Geometry check sheet. Reference: the model listing, model coordinates, mm. A direction names the side the tool comes from. Give positions to 0.01 mm unless a question says otherwise; leave off trailing zeros. Loops run counter-clockwise (first coordinate to the right, second up) from the corner with the lowest first, then second, coordinate; pieces in that order, holes last. Notation, with made-up numbers: (-17.75, 75) -> (-9.75, 75) arc R4 ccw to (-9.75, 82) -> close; hole circle Ø5 at (45, 63). An arc over 180 degrees is marked (long way). Answer in a Markdown table with one row per item. Add a question column.
```python
from build123d import *

# Parameters (mm, degrees)
SKETCH1_W                 = 146.5
SKETCH1_H                 = 20
BOSS_EXTRUDE1_DEPTH       = 2
SKETCH2_W                 = 10
SKETCH2_H                 = 1
BOSS_EXTRUDE2_DEPTH       = 60
SKETCH3_W                 = 20
SKETCH3_H                 = 1
BOSS_EXTRUDE3_DEPTH       = 3
SKETCH4_W                 = 20
SKETCH4_H                 = 1
BOSS_EXTRUDE4_DEPTH       = 3
BOSS_EXTRUDE5_DEPTH       = 3
BOSS_EXTRUDE5_DEPTH_BACK  = 13
SKETCH5_W                 = 20
SKETCH5_H                 = 1
BOSS_EXTRUDE7_DEPTH       = 3
BOSS_EXTRUDE7_DEPTH_BACK  = 13
SKETCH7_W                 = 20
SKETCH7_H                 = 1
BOSS_EXTRUDE9_DEPTH       = 3
BOSS_EXTRUDE9_DEPTH_BACK  = 13
SKETCH9_W                 = 20
SKETCH9_H                 = 1
BOSS_EXTRUDE11_DEPTH      = 3
BOSS_EXTRUDE11_DEPTH_BACK = 13
SKETCH11_W                = 20
SKETCH11_H                = 1
SKETCH13_W                = 30
SKETCH13_H                = 1
BOSS_EXTRUDE13_DEPTH      = 3
SKETCH14_W                = 20
SKETCH14_H                = 1
BOSS_EXTRUDE14_DEPTH      = 3
CUT_EXTRUDE1_DEPTH        = 3
SKETCH16_W                = 5
SKETCH16_H                = 20
CUT_EXTRUDE2_DEPTH        = 10
SKETCH17_W                = 5
SKETCH17_H                = 40
SKETCH17_W_2              = 8
CUT_EXTRUDE3_DEPTH        = 10
FILLET1_R                 = 3
FILLET2_R                 = 2.5


with BuildPart() as part:
    # Sketch1 → Boss-Extrude1 (new body)
    with BuildSketch(Plane.XY):
        with Locations((-1709.906073211, 816.567138103)):
            Rectangle(SKETCH1_W, SKETCH1_H)
    extrude(amount=BOSS_EXTRUDE1_DEPTH)

    # Sketch2 → Boss-Extrude2 (add)
    with BuildSketch(Plane.XY.offset(2)):
        with Locations((-1778.156073211, 826.067138103)):
            Rectangle(SKETCH2_W, SKETCH2_H)
        with Locations((-1754.656073211, 826.067138103)):
            Rectangle(SKETCH2_W, SKETCH2_H)
        with Locations((-1641.656073211, 826.067138103)):
            Rectangle(SKETCH2_W, SKETCH2_H)
        with Locations((-1665.156073211, 826.067138103)):
            Rectangle(SKETCH2_W, SKETCH2_H)
        with Locations((-1721.656073211, 826.067138103)):
            Rectangle(SKETCH2_W, SKETCH2_H)
        with Locations((-1698.156073211, 826.067138103)):
            Rectangle(SKETCH2_W, SKETCH2_H)
    extrude(amount=BOSS_EXTRUDE2_DEPTH)

    # Sketch3 → Boss-Extrude3 (add)
    with BuildSketch(Plane.ZY.offset(1783.156073211)):
        with Locations((52, 826.067138103)):
            Rectangle(SKETCH3_W, SKETCH3_H)
    extrude(amount=BOSS_EXTRUDE3_DEPTH)

    # Sketch4 → Boss-Extrude4 (add)
    with BuildSketch(Plane(origin=(-1773.156073211, 0, 0), x_dir=(0, 0, -1), z_dir=(1, 0, 0))):
        with Locations((-52, 826.067138104)):
            Rectangle(SKETCH4_W, SKETCH4_H)
    extrude(amount=BOSS_EXTRUDE4_DEPTH)

    # Sketch5 → Boss-Extrude5 (add, two sides: drawn at the far end of the back side and taken through both)
    with BuildSketch(Plane.ZY.offset(1759.656073211).offset(-BOSS_EXTRUDE5_DEPTH_BACK)):
        with Locations((52, 826.067138103)):
            Rectangle(SKETCH5_W, SKETCH5_H)
    extrude(amount=BOSS_EXTRUDE5_DEPTH + BOSS_EXTRUDE5_DEPTH_BACK)

    # Sketch7 → Boss-Extrude7 (add, two sides: drawn at the far end of the back side and taken through both)
    with BuildSketch(Plane.ZY.offset(1726.656073211).offset(-BOSS_EXTRUDE7_DEPTH_BACK)):
        with Locations((52, 826.067138103)):
            Rectangle(SKETCH7_W, SKETCH7_H)
    extrude(amount=BOSS_EXTRUDE7_DEPTH + BOSS_EXTRUDE7_DEPTH_BACK)

    # Sketch9 → Boss-Extrude9 (add, two sides: drawn at the far end of the back side and taken through both)
    with BuildSketch(Plane.ZY.offset(1703.156073211).offset(-BOSS_EXTRUDE9_DEPTH_BACK)):
        with Locations((52, 826.067138103)):
            Rectangle(SKETCH9_W, SKETCH9_H)
    extrude(amount=BOSS_EXTRUDE9_DEPTH + BOSS_EXTRUDE9_DEPTH_BACK)

    # Sketch11 → Boss-Extrude11 (add, two sides: drawn at the far end of the back side and taken through both)
    with BuildSketch(Plane.ZY.offset(1670.156073211).offset(-BOSS_EXTRUDE11_DEPTH_BACK)):
        with Locations((52, 826.067138103)):
            Rectangle(SKETCH11_W, SKETCH11_H)
    extrude(amount=BOSS_EXTRUDE11_DEPTH + BOSS_EXTRUDE11_DEPTH_BACK)

    # Sketch13 → Boss-Extrude13 (add)
    with BuildSketch(Plane(origin=(-1636.656073211, 0, 0), x_dir=(0, 0, -1), z_dir=(1, 0, 0))):
        with Locations((-47, 826.067138103)):
            Rectangle(SKETCH13_W, SKETCH13_H)
    extrude(amount=BOSS_EXTRUDE13_DEPTH)

    # Sketch14 → Boss-Extrude14 (add)
    with BuildSketch(Plane.ZY.offset(1646.656073212)):
        with Locations((52, 826.067138102)):
            Rectangle(SKETCH14_W, SKETCH14_H)
    extrude(amount=BOSS_EXTRUDE14_DEPTH)

    # Sketch15 → Cut-Extrude1 (cut)
    with BuildSketch(Plane.XY.offset(2)):
        with BuildLine():
            Line((-1711.506073211, 810.067138103), (-1711.506073211, 823.067138103))
            ThreePointArc((-1711.506073211, 823.067138103), (-1709.906073211, 824.667138103), (-1708.306073211, 823.067138103))
            Line((-1708.306073211, 823.067138103), (-1708.306073211, 810.067138103))
            ThreePointArc((-1708.306073211, 810.067138103), (-1709.906073211, 808.467138103), (-1711.506073211, 810.067138103))
        make_face()
    extrude(amount=-CUT_EXTRUDE1_DEPTH, mode=Mode.SUBTRACT)

    # Sketch16 → Cut-Extrude2 (cut)
    with BuildSketch(Plane.XY.offset(2)):
        with Locations((-1780.656073211, 816.567138103)):
            Rectangle(SKETCH16_W, SKETCH16_H)
        with Locations((-1639.156073211, 816.567138103)):
            Rectangle(SKETCH16_W, SKETCH16_H)
    extrude(amount=-CUT_EXTRUDE2_DEPTH, mode=Mode.SUBTRACT)

    # Sketch17 → Cut-Extrude3 (cut)
    with BuildSketch(Plane.XZ.offset(-825.567138103)):
        with Locations((-1780.656073211, 22)):
            Rectangle(SKETCH17_W, SKETCH17_H)
        with Locations((-1637.656073211, 22)):
            Rectangle(SKETCH17_W_2, SKETCH17_H)
    extrude(amount=-CUT_EXTRUDE3_DEPTH, mode=Mode.SUBTRACT)

    # Fillet1
    fillet1_edges = [part.edges().sort_by_distance(p)[0] for p in [
        (-1775.656073211, 825.567138103, 2),
        (-1644.156073211, 825.567138103, 2),
    ]]
    fillet(fillet1_edges, radius=FILLET1_R)

    # Fillet2
    fillet2_edges = [part.edges().sort_by_distance(p)[0] for p in [
        (-1754.656073211, 825.567138103, 2),
        (-1665.156073211, 825.567138103, 2),
        (-1721.656073211, 825.567138103, 2),
        (-1698.156073211, 825.567138103, 2),
    ]]
    fillet(fillet2_edges, radius=FILLET2_R)


solid = part.part
```
1. Gauge pin test, flat ends, axial feed: pin 1 Ø1.8 at (y, z) = (825.5, 13.5) entering from -X; pin 2 Ø0.5 at (x, y) = (-1638, 826) entering from -Z; pin 3 Ø5 at (x, z) = (-1754, 26) entering from -Y; pin 4 Ø1.8 at (y, z) = (824.5, 12) entering from +X. Record the tip position at first contact, or that the pin passes through.
2. Sectioned sample at C-C (z = 20.5). Enter the section's corners in (x, y).
3. Access from +Z, -Z, +X, -X, +Y, -Y to the whole of each face (thin tool, end or side, straight path). Record for faces 4 (the face through (-1665.1, 824.9, 2.8)), 5 (the face through (-1646.656, 826, 22)), 6 (the face through (-1698, 825.567, 39)), 7 (the face through (-1726, 826.567, 37)).
4. Material ranges on L1, parallel to Z at x = -1747, y = 811.75; L2, parallel to Y at x = -1753.5, z = 14; L3, parallel to Z at x = -1780, y = 826, recorded low to high. Write a range as from..to.
5. Sectioned sample at B-B (y = 819). Enter the section's corners in (x, z), plus the area to 3 significant figures.
6. Release check for a two-part mould opening along X. For faces 1 (the face through (-1726.656, 826, 20)), 2 (the face through (-1722, 825.567, 39)), 3 (the face through (-1641.656, 826, 10)) record: released by +X, released by -X, zero draft, split by the parting line, or undercut.
7. Sectioned sample at A-A (z = 47). Enter the section's corners in (x, y), plus the area to 3 significant figures.
8. Sectioned sample at D-D (x = -1733). Enter the section's corners in (y, z), plus the area to 3 significant figures.
Response:
| question | item | result |
|---|---|---|
| 1 | pin 1 | stops at x = -1778.16 |
| 1 | pin 2 | stops at z = 42 |
| 1 | pin 3 | stops at y = 825.57 |
| 1 | pin 4 | passes through |
| 2 | outline | (-1778.16, 825.57) -> (-1773.16, 825.57) -> (-1773.16, 826.57) -> (-1778.16, 826.57) -> close; (-1759.66, 825.57) -> (-1749.66, 825.57) -> (-1749.66, 826.57) -> (-1759.66, 826.57) -> close; (-1726.66, 825.57) -> (-1716.66, 825.57) -> (-1716.66, 826.57) -> (-1726.66, 826.57) -> close; (-1703.16, 825.57) -> (-1693.16, 825.57) -> (-1693.16, 826.57) -> (-1703.16, 826.57) -> close; (-1670.16, 825.57) -> (-1660.16, 825.57) -> (-1660.16, 826.57) -> (-1670.16, 826.57) -> close; (-1646.66, 825.57) -> (-1641.66, 825.57) -> (-1641.66, 826.57) -> (-1646.66, 826.57) -> close |
| 3 | face 4 | +Z, -Y |
| 3 | face 5 | +Y, -Y |
| 3 | face 6 | +Z, +X, -X, -Y |
| 3 | face 7 | +Z, -Z, +X, -X, +Y |
| 4 | L1 | z = 0..2 |
| 4 | L2 | y = 825.57..826.57 |
| 4 | L3 | z = 42..62 |
| 5 | outline | (-1778.16, 0) -> (-1711.51, 0) -> (-1711.51, 2) -> (-1778.16, 2) -> close; (-1708.31, 0) -> (-1641.66, 0) -> (-1641.66, 2) -> (-1708.31, 2) -> close |
| 5 | area | 267 mm2 |
| 6 | face 1 | undercut |
| 6 | face 2 | zero draft |
| 6 | face 3 | released by +X |
| 7 | outline | (-1786.16, 825.57) -> (-1770.16, 825.57) -> (-1770.16, 826.57) -> (-1786.16, 826.57) -> close; (-1762.66, 825.57) -> (-1746.66, 825.57) -> (-1746.66, 826.57) -> (-1762.66, 826.57) -> close; (-1729.66, 825.57) -> (-1713.66, 825.57) -> (-1713.66, 826.57) -> (-1729.66, 826.57) -> close; (-1706.16, 825.57) -> (-1690.16, 825.57) -> (-1690.16, 826.57) -> (-1706.16, 826.57) -> close; (-1673.16, 825.57) -> (-1657.16, 825.57) -> (-1657.16, 826.57) -> (-1673.16, 826.57) -> close; (-1649.66, 825.57) -> (-1633.66, 825.57) -> (-1633.66, 826.57) -> (-1649.66, 826.57) -> close |
| 7 | area | 96.0 mm2 |
| 8 | outline | (806.57, 0) -> (826.57, 0) -> (826.57, 2) -> (806.57, 2) -> close |
| 8 | area | 40.0 mm2 |
